```python
from build123d import *

# Parameters (mm, degrees)
CUFF_STOPPER_SKETCH_R                 = 30
CUFF_STOPPER_EXTRUDE_DEPTH            = 5
CUFF_PIN_SKETCH_R                     = 10
CUFF_PIN_EXTRUDE_DEPTH                = 42
SUPPORT_SKETCH_W                      = 40
SUPPORT_SKETCH_H                      = 40
SUPPORT_EXTRUDE_DEPTH                 = 25
PIN_SUPPORT_EXTRUDE_REACH             = 61.699
PIN_SUPPORT_EXTRUDE_DIRECTION_2_REACH = 61.699
PIN_HOLE_SKETCH_R                     = 10
PIN_HOLE_CUT_DEPTH                    = 40


with BuildPart() as part:
    # Cuff Stopper Sketch → Cuff Stopper Extrude (new body)
    with BuildSketch(Plane.XY):
        Circle(CUFF_STOPPER_SKETCH_R)
    extrude(amount=-CUFF_STOPPER_EXTRUDE_DEPTH)

    # Cuff Pin Sketch → Cuff Pin Extrude (add)
    with BuildSketch(Plane.XY):
        with Locations(Location((0, 0, 0), (0, 0, 180))):
            Circle(CUFF_PIN_SKETCH_R)
    extrude(amount=CUFF_PIN_EXTRUDE_DEPTH)

    # Support Sketch → Support Extrude (add)
    with BuildSketch(Plane(origin=(0, 0, -5), x_dir=(-1, 0, 0), z_dir=(0, 0, -1))):
        Rectangle(SUPPORT_SKETCH_W, SUPPORT_SKETCH_H)
    extrude(amount=SUPPORT_EXTRUDE_DEPTH)

    # Pin Support Extrude: up to this face of the body (flat: up to its plane)
    pin_support_extrude_end = Plane(part.part.faces().sort_by_distance((0, 20, -17.5))[0])
    # Pin Support Sketch → Pin Support Extrude (add, up to the picked face)
    with BuildSketch(Plane(origin=(0, 0, 0), x_dir=(1, 0, 0), z_dir=(0, 1, 0)), mode=Mode.PRIVATE) as pin_support_extrude_sk1:
        with BuildLine():
            Line((20, 30), (-20, 30))
            ThreePointArc((-20, 30), (0, 50), (20, 30))
        make_face()
    pin_support_extrude_tool1 = split(extrude(pin_support_extrude_sk1.sketch, amount=PIN_SUPPORT_EXTRUDE_REACH, mode=Mode.PRIVATE), bisect_by=pin_support_extrude_end, keep=Keep.BOTH, mode=Mode.PRIVATE)
    add(pin_support_extrude_tool1.solids().sort_by(Axis((0, 0, -38.488264), (0, 1, 0)))[0])

    # Pin Support Extrude direction 2: up to this face of the body (flat: up to its plane)
    pin_support_extrude_direction_2_end = Plane(part.part.faces().sort_by_distance((0, -20, -17.5))[0])
    # Pin Support Sketch → Pin Support Extrude direction 2 (add, up to the picked face)
    with BuildSketch(Plane(origin=(0, 0, 0), x_dir=(1, 0, 0), z_dir=(0, 1, 0)), mode=Mode.PRIVATE) as pin_support_extrude_direction_2_sk1:
        with BuildLine():
            Line((20, 30), (-20, 30))
            ThreePointArc((-20, 30), (0, 50), (20, 30))
        make_face()
    pin_support_extrude_direction_2_tool1 = split(extrude(pin_support_extrude_direction_2_sk1.sketch, amount=-PIN_SUPPORT_EXTRUDE_DIRECTION_2_REACH, mode=Mode.PRIVATE), bisect_by=pin_support_extrude_direction_2_end, keep=Keep.BOTH, mode=Mode.PRIVATE)
    add(pin_support_extrude_direction_2_tool1.solids().sort_by(Axis((0, 0, -38.488264), (0, -1, 0)))[0])

    # Pin Hole Sketch → Pin Hole Cut (cut)
    with BuildSketch(Plane(origin=(0, 20, 0), x_dir=(1, 0, 0), z_dir=(0, 1, 0))):
        with Locations(Location((0, 30, 0), (0, 0, 270))):
            Circle(PIN_HOLE_SKETCH_R)
    extrude(amount=-PIN_HOLE_CUT_DEPTH, mode=Mode.SUBTRACT)


solid = part.part
```
Here's how the part is built. I have some questions about the finished solid (model axes, mm). A direction names the side the tool comes from. Coordinates: 2 decimals unless noted, no trailing zeros. Order: outer loops, then holes, each group sorted by start corner. A loop starts at its lowest first (then second) coordinate and runs counter-clockwise, first axis right, second up.
Item 1: If we section it at A-A, the plane x = 0: List the corners of the cut face in (y, z) for me, then the cut area to 3 significant figures.
Response values:
outline: (-30, -5) - (-20, -5) - (-20, -20) - (20, -20) - (20, -5) - (30, -5) - (30, 0) - (10, 0) - (10, 42) - (-10, 42) - (-10, 0) - (-30, 0) - close; (-20, -50) - (20, -50) - (20, -40) - (-20, -40) - close
area: 2,140 mm2
Item 2: If we section it at D-D, the plane x = -18.5: List the corners of the cut face in (y, z) for me, then the cut area to 3 significant figures.
Response values:
outline: (-23.62, -5) - (-20, -5) - (-20, -37.6) - (20, -37.6) - (20, -5) - (23.62, -5) - (23.62, 0) - (-23.62, 0) - close
area: 1,540 mm2
Item 3: I'm going to push flat-ended pins straight in: pin 1 Ø12 at (y, z) = (-13, 19.5) entering from -X; pin 2 Ø12 at (x, z) = (-11, 5) entering from -Y; pin 3 Ø8 at (y, z) = (3.5, -15.5) entering from +X. Where does each tip first touch, or does it pass through?
Response values:
pin 1: stops at x = -7.14
pin 2: stops at y = -29
pin 3: stops at x = 20
Item 4: I need wall thicknesses on probe 1 along X at (y, z) = (3.5, -30); probe 2 along X at (y, z) = (5, -10.5). Which ranges of each line are inside material? Lowest first, please.
Response values:
probe 1: x = -20 to -10, 10 to 20
probe 2: x = -20 to 20
Item 5: If we section it at B-B, the plane y = 0: List the corners of the cut face in (x, z) for me.
Response values:
outline: (-30, -5) - (-20, -5) - (-20, -30) arc R20 ccw to (20, -30) - (20, -5) - (30, -5) - (30, 0) - (10, 0) - (10, 42) - (-10, 42) - (-10, 0) - (-30, 0) - close; hole circle Ø20 at (0, -30)
Item 6: If we section it at C-C, the plane z = -33.5: List the corners of the cut face in (x, y) for me, then the cut area to 3 significant figures.
Response values:
outline: (-19.69, -20) - (-9.37, -20) - (-9.37, 20) - (-19.69, 20) - close; (9.37, -20) - (19.69, -20) - (19.69, 20) - (9.37, 20) - close
area: 826 mm2
Item 7: Thinking about a two-plate mould opening in Z: for faces 5 (the face through (20, 0, -17)), 6 (the face through (0, 0, -50)), 7 (the face through (13, 0, 0)), 8 (the face through (0, 0, -40)), which applies, pulls with the +Z half, pulls with the -Z half, needs draft (parallel to the pull), parting line crosses it, or undercut?
Response values:
face 5: needs draft
face 6: pulls with the -Z half
face 7: pulls with the +Z half
face 8: undercut
Item 8: Which directions (+Z, -Z, +X, -X, +Y, -Y) give clear straight access to the entire face, cutting with the end or side of a thin tool? Please do faces 1 (the face through (10, 0, 21)), 2 (the face through (-20, 0, -17)), 3 (the face through (0, 20, -17)), 4 (the face through (0, -20, -18)).
Response values:
face 1: +Z
face 2: -Z, -X, +Y, -Y
face 3: -Z, +X, -X, +Y
face 4: -Z, +X, -X, -Y
